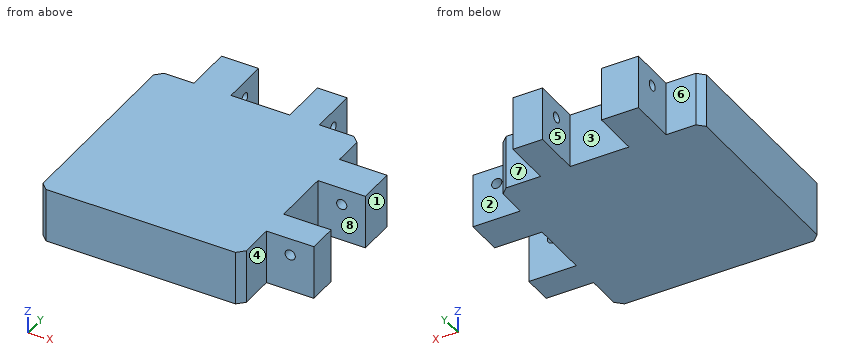
Autodesk Inventor part; units mm, degrees
ref_plane "YZ Plane" through (0, 0, 0) normal (1, 0, 0) x (0, 1, 0)
ref_plane "XZ Plane" through (0, 0, 0) normal (0, 1, 0) x (-1, 0, 0)
ref_plane "XY Plane" through (0, 0, 0) normal (0, 0, 1) x (1, 0, 0)
ref_plane "Work Plane1" through (0, 0, 0) normal (0, 0, 1) x (1, 0, 0)
sketch "Sketch1" plane through (0, 0, 0) normal (0, 0, 1) x (1, 0, 0)
  circle A0 centre (17.5, 17.5) radius 1.95
  circle A1 centre (17.5, -17.5) radius 1.95
  circle A2 centre (-17.5, -17.5) radius 1.95
  circle A3 centre (-17.5, 17.5) radius 1.95
  circle A4 centre (0, 0) radius 7.5
  line L0 (-30, 28) -> (-28, 30)
  line L1 (-30, -28) -> (-30, 28)
  line L2 (-28, -30) -> (-30, -28)
  line L3 (28, -30) -> (-28, -30)
  line L4 (30, -28) -> (28, -30)
  line L5 (30, 28) -> (30, -28)
  line L6 (28, 30) -> (30, 28)
  line L7 (-28, 30) -> (28, 30)
  circle A5 centre (25, 25) radius 2.325
  circle A6 centre (-25, -25) radius 2.325
  circle A7 centre (25, -25) radius 2.325
  circle A8 centre (-25, 25) radius 2.325
  circle A9 centre (10, -25) radius 1.45
  circle A10 centre (10, 25) radius 1.45
  circle A11 centre (-10, 25) radius 1.45
  circle A12 centre (-10, -25) radius 1.45
  circle A13 centre (-25, -10) radius 1.45
  circle A14 centre (25, -10) radius 1.45
  circle A15 centre (25, 10) radius 1.45
  circle A16 centre (-25, 10) radius 1.45
  point P0 (0, 0)
extrude "Extrusion1" add sketch "Sketch1" along normal blind 16 contours A0 | A1 | A2 | A3 | A4 | L0 L7 L6 L5 L4 L3 L2 L1 | A5 | A6 | A7 | A8 | A9 | A10 | A11 | A12 | A13 | A14 | A15 | A16
sketch "Sketch2" plane through (0, 0, 16) normal (0, 0, 1) x (1, 0, 0)
  point P0 (0, 0)
sketch "Sketch3" plane through (30, -28, 0) normal (1, 0, 0) x (0, 0, -1)
  line L0 (0, 56) -> (0, 0)
  line L1 (0, 56) -> (-16, 56)
  line L2 (-16, 0) -> (-16, 56)
  line L3 (0, 0) -> (-16, 0)
  line L4 (-16, 0) -> (-16, 56)
  line L5 (0, 47.2331) -> (-16, 47.2331)
  line L6 (-16, 47.2331) -> (-16, 36.3051)
  line L7 (-16, 36.3051) -> (0, 36.3051)
  line L8 (0, 36.3051) -> (0, 47.2331)
  line L9 (0, 56) -> (0, 0)
  line L10 (0, 10.2066) -> (-16, 10.2066)
  line L11 (-16, 10.2066) -> (-16, 18.9489)
  line L12 (-16, 18.9489) -> (0, 18.9489)
  line L13 (0, 18.9489) -> (0, 10.2066)
  point P0 (0, 28)
extrude "Extrusion2" add sketch "Sketch3" along normal blind 14 contours L0 L7 L2 L5 | L0 L10 L2 L12
sketch "Sketch4" plane through (30, 19.2331, 16) normal (0, 1, 0) x (1, 0, 0)
  line L0 (0, 0) -> (0, 16)
  line L1 (0, 0) -> (14, 0)
  line L2 (14, 16) -> (14, 0)
  line L3 (0, 16) -> (14, 16)
  circle A0 centre (7, 5) radius 1.5
  point P0 (-30, 16)
  dimension "d4" = 3
extrude "Extrusion3" cut sketch "Sketch4" against normal through all contours A0
pattern_circular "Circular Pattern1" count 2 over 90 about axis through (0, 0, 0) along (0, 0, 1) of "Extrusion2", "Extrusion3"
properties part number "00_XY_stage-CHUO_SEIKI_LD-647-R1-Middle"
For this review, take the finished solid that the model builds, in its own axes (mm). Face numbers are marked on the shaded views. A direction names the side the tool comes from. Give positions to 0.01 mm unless a question says otherwise; leave off trailing zeros. Order: outer loops, then holes, each group sorted by start corner. A loop starts at its lowest first (then second) coordinate and runs counter-clockwise, first axis right, second up. Notation, with made-up numbers: (6, -40) -> (27, -40) arc R26 cw to (27, -8) -> close; hole circle Ø11 at (73, 1). An arc over 180 degrees is marked (long way). Write item = value, one per line.
1) We need section C-C, the plane z = 14.5. Give the boundary of the cut face in (x, y).
Findings:
outline = (-30, -28) -> (-28, -30) -> (28, -30) -> (30, -28) -> (30, -17.79) -> (44, -17.79) -> (44, -9.05) -> (30, -9.05) -> (30, 8.31) -> (44, 8.31) -> (44, 19.23) -> (30, 19.23) -> (30, 28) -> (28, 30) -> (17.79, 30) -> (17.79, 44) -> (9.05, 44) -> (9.05, 30) -> (-8.31, 30) -> (-8.31, 44) -> (-19.23, 44) -> (-19.23, 30) -> (-28, 30) -> (-30, 28) -> close
2) Draft analysis for pull direction X (two halves, no side actions). For the marked faces 1, 2 and 3, state which applies: pulls with the +X half, pulls with the -X half, needs draft (parallel to the pull), parting line crosses it, or undercut.
Findings:
face_1 = pulls with the +X half
face_2 = needs draft
face_3 = undercut
3) To check wall thickness, follow L1, parallel to X at y = 32.5, z = 4.25; L2, parallel to X at y = 16.5, z = 11. State the ranges of each line that lie inside material, in increasing order. Write a range as from..to.
Findings:
L1 = -19.23..-8.31, 9.05..17.79
L2 = -30..35.5, 38.5..44
4) Insertion check: pin 1 (7 mm diameter, centred on y = 34.5, z = 10.5, fed in from -X); pin 2 (4 mm diameter, centred on y = 40, z = 5.5, fed in from +X); pin 3 (2.5 mm diameter, centred on x = -25.5, z = 6, fed in from +Y). Each pin has a flat end and moves straight along its axis. Give the tip position at first contact, or say it passes through.
Findings:
pin_1 = -19.23
pin_2 = 17.79
pin_3 = 30
5) We need section A-A, the plane y = 37. Give the boundary of the cut face in (x, z), and give its area (3 significant figures).
Findings:
outline = (-19.23, 0) -> (-8.31, 0) -> (-8.31, 9.5) -> (-19.23, 9.5) -> close; (-19.23, 12.5) -> (-8.31, 12.5) -> (-8.31, 16) -> (-19.23, 16) -> close; (9.05, 0) -> (17.79, 0) -> (17.79, 9.5) -> (9.05, 9.5) -> close; (9.05, 12.5) -> (17.79, 12.5) -> (17.79, 16) -> (9.05, 16) -> close
area = 256 mm^2
6) We need section B-B, the plane x = 37. Give the boundary of the cut face in (y, z).
Findings:
outline = (-17.79, 0) -> (-9.05, 0) -> (-9.05, 9.5) -> (-17.79, 9.5) -> close; (-17.79, 12.5) -> (-9.05, 12.5) -> (-9.05, 16) -> (-17.79, 16) -> close; (8.31, 0) -> (19.23, 0) -> (19.23, 9.5) -> (8.31, 9.5) -> close; (8.31, 12.5) -> (19.23, 12.5) -> (19.23, 16) -> (8.31, 16) -> close
7) We need section D-D, the plane x = 7.5. Give the boundary of the cut face in (y, z), and give its area (3 significant figures).
Findings:
outline = (-30, 0) -> (30, 0) -> (30, 16) -> (-30, 16) -> close
area = 960 mm^2
8) For the marked faces 4, 5, 6, 7 and 8, list the 3-axis set-ups (+Z, -Z, +X, -X, +Y, -Y) from which the entire face can be reached by the end or side of a thin tool; tool diameter is ignored.
Findings:
face_4 = +Z, -Z, +X, -Y
face_5 = +Z, -Z, +Y
face_6 = +Z, -Z, -X, +Y
face_7 = +Z, -Z, +X, +Y
face_8 = +Z, -Z, +X
